Could you check a few things on this model? Use its own coordinates, in mm. Face numbers are marked on the shaded views. A direction names the side the tool comes from. Round coordinates to 2 decimals unless told otherwise and drop trailing zeros. Write each loop counter-clockwise with the first axis right and the second up, starting at its lowest first coordinate (ties: lowest second). Pieces come first, ordered by that corner, then holes. Notation, with made-up numbers: (34.25, 79.25) -> (39.25, 79.25) arc R23 ccw to (39.25, 109.25) -> close; hole circle Ø1 at (15.25, 81). An arc over 180 degrees is marked (long way). Answer in a Markdown table with one row per item. Add a question column.
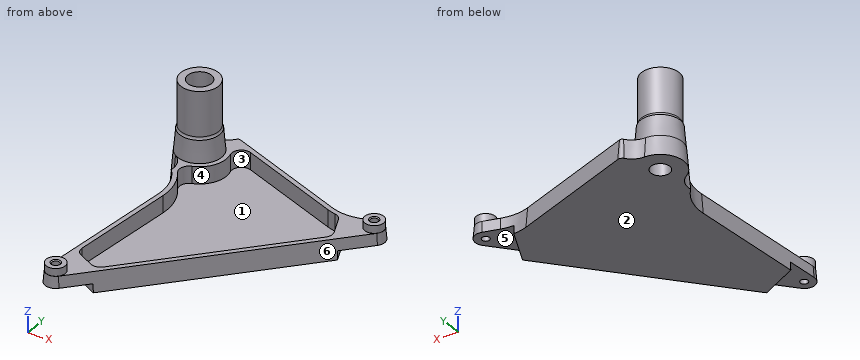
```python
from build123d import *
from build123d.topology import SkipClean

# Parameters (mm, degrees)
EXTRUDE_741_DEPTH      = 21
EXTRUDE_741_TAPER      = 5
SKETCH_2_R             = 10
EXTRUDE_1024_DEPTH     = 8
CUT_EXTRUDE_1617_DEPTH = 9
SKETCH_4_R             = 23.162738066
EXTRUDE_1852_DEPTH     = 23
EXTRUDE_1852_TAPER     = 5
SKETCH_5_R             = 20
EXTRUDE_1938_DEPTH     = 50
FILLET_1977_R          = 4
SKETCH_6_R             = 12.5
CUT_EXTRUDE_2083_DEPTH = 24
SKETCH_7_R             = 10
CUT_EXTRUDE_2165_DEPTH = 330.802615362
FILLET_2203_R          = 0.3
SKETCH_8_R             = 4
CUT_EXTRUDE_2369_DEPTH = 329.777683375
CHAMFER_2404_SIZE      = 1
CUT_EXTRUDE_3109_DEPTH = 18


with BuildPart() as part:
    # Эскиз1 → Extrude 741 (new body)
    with BuildSketch(Plane.XY):
        with BuildLine():
            ThreePointArc((206.902825712, -28.037707575), (208.16042902, -13.627270923), (194.643197369, -8.47686326))
            Line((194.643197369, -8.47686326), (178.352602864, -13.211762774))
            ThreePointArc((178.352602864, -13.211762774), (164.281318134, -14.974601832), (150.3601632, -12.270882024))
            Line((150.3601632, -12.270882024), (21.714759937, 34.696764669))
            ThreePointArc((21.714759937, 34.696764669), (18.576858011, 34.793189635), (16, 33))
            ThreePointArc((16, 33), (8.94427191, 27.11145618), (0, 25))
            ThreePointArc((0, 25), (-24.017605322, 6.939354046), (-13.333333333, -21.147629234))
            ThreePointArc((-13.333333333, -21.147629234), (-5.735545873, -29.916516988), (-4.284649798, -41.428018512))
            ThreePointArc((-4.284649798, -41.428018512), (6.155658081, -59.36704661), (8.411759167, -80))
            Line((8.411759167, -80), (-6.939849245, -232.746575098))
            ThreePointArc((-6.939849245, -232.746575098), (0.139115456, -244.91798346), (13.910401615, -241.984282673))
            Line((13.910401615, -241.984282673), (206.902825712, -28.037707575))
        make_face()
    extrude(amount=EXTRUDE_741_DEPTH, taper=EXTRUDE_741_TAPER)

    # Эскиз2 → Extrude 1024 (add)
    with BuildSketch(Plane.XY.offset(21)):
        with Locations((5, -233.946575098)):
            Circle(SKETCH_2_R)
        with Locations((197.992424097, -20)):
            Circle(SKETCH_2_R)
    extrude(amount=EXTRUDE_1024_DEPTH)

    # Эскиз3 → Cut-Extrude 1617 (cut)
    with BuildSketch(Plane(origin=(0, 0, 0), x_dir=(-1, 0, 0), z_dir=(0, 0, -1))):
        with BuildLine():
            Line((-164.992424097, -14.992878037), (-182.581248366, -55))
            Line((-182.581248366, -55), (-206.902825712, -28.037707575))
            ThreePointArc((-206.902825712, -28.037707575), (-208.364208989, -13.964597929), (-195.406790483, -8.281873067))
            Line((-195.406790483, -8.281873067), (-164.992424097, -14.992878037))
        make_face()
        with BuildLine():
            Line((3.643325211, -199.946575098), (-34.691772051, -218.946575098))
            Line((-34.691772051, -218.946575098), (-13.910401615, -241.984282673))
            ThreePointArc((-13.910401615, -241.984282673), (-0.139115456, -244.91798346), (6.939849245, -232.746575098))
            Line((6.939849245, -232.746575098), (3.643325211, -199.946575098))
        make_face()
    extrude(amount=-CUT_EXTRUDE_1617_DEPTH, mode=Mode.SUBTRACT)

    # Эскиз4 → Extrude 1852 (add)
    with SkipClean():  # the faces are left unmerged after this step: merging them gives an invalid solid
        with BuildSketch(Plane.XY.offset(21)):
            Circle(SKETCH_4_R)
        extrude(amount=EXTRUDE_1852_DEPTH, taper=EXTRUDE_1852_TAPER)

    # Эскиз5 → Extrude 1938 (add)
    with SkipClean():  # the faces are left unmerged after this step: merging them gives an invalid solid
        with BuildSketch(Plane.XY.offset(44)):
            Circle(SKETCH_5_R)
        extrude(amount=EXTRUDE_1938_DEPTH)

    # Fillet 1977
    # the kernel refuses this fillet: 4 mm, written as the material it adds along each edge
    with BuildSketch(Plane(origin=(0, 0, 44), x_dir=(1, 0, 0), z_dir=(0, -1, 0))) as fillet_1977_piece_1:
        with BuildLine():
            CenterArc((24, 2.807194852), FILLET_1977_R, 180, 44.571493735)
            Line((20, 2.807194852), (19.92, 2.807194852))
            Line((19.92, 2.807194852), (19.92, 0))
            Line((19.92, 0), (20, -0.08))
            ThreePointArc((20, -0.08), (20.575249402, -0.08), (21.093508781, -0.056143897))
            Line((21.093508781, -0.056143897), (21.150498805, 0))
        make_face()
    revolve(axis=Axis((0, 0, 44), (0, 0, 1)))

    # Эскиз6 → Cut-Extrude 2083 (cut)
    with SkipClean():  # the faces are left unmerged after this step: merging them gives an invalid solid
        with BuildSketch(Plane.XY.offset(94)):
            Circle(SKETCH_6_R)
        extrude(amount=-CUT_EXTRUDE_2083_DEPTH, mode=Mode.SUBTRACT)

    # Эскиз7 → Cut-Extrude 2165 (cut, through all)
    with SkipClean():  # the faces are left unmerged after this step: merging them gives an invalid solid
        with BuildSketch(Plane.XY.offset(70)):
            Circle(SKETCH_7_R)
        extrude(amount=-CUT_EXTRUDE_2165_DEPTH, mode=Mode.SUBTRACT)

    # Fillet 2203
    fillet_2203_edges = [part.edges().sort_by_distance(p)[0] for p in [
        (-10, 0, 70),
    ]]
    fillet(fillet_2203_edges, radius=FILLET_2203_R)

    # Эскиз8 → Cut-Extrude 2369 (cut, through all)
    with SkipClean():  # the faces are left unmerged after this step: merging them gives an invalid solid
        with BuildSketch(Plane.XY.offset(29)):
            with Locations((197.992424097, -20)):
                Circle(SKETCH_8_R)
            with Locations((5, -233.946575098)):
                Circle(SKETCH_8_R)
        extrude(amount=-CUT_EXTRUDE_2369_DEPTH, mode=Mode.SUBTRACT)

    # Chamfer 2404
    chamfer_2404_edges = [part.edges().sort_by_distance(p)[0] for p in [
        (193.992424097, -20, 29),
        (1, -233.946575098, 29),
    ]]
    chamfer(chamfer_2404_edges, length=CHAMFER_2404_SIZE)

    # Эскиз11 → Cut-Extrude 3109 (cut)
    with SkipClean():  # the faces are left unmerged after this step: merging them gives an invalid solid
        with BuildSketch(Plane.XY.offset(21)):
            with BuildLine():
                Line((9.637769662, -200.948644603), (25.017172577, -208.571128339))
                ThreePointArc((25.017172577, -208.571128339), (31.330335402, -209.434392448), (36.883287498, -206.3093368))
                Line((36.883287498, -206.3093368), (171.559935828, -57.010172388))
                ThreePointArc((171.559935828, -57.010172388), (174.007077586, -51.904002649), (173.288958057, -46.287439952))
                Line((173.288958057, -46.287439952), (164.797960407, -26.974018349))
                ThreePointArc((164.797960407, -26.974018349), (161.780560792, -23.10323492), (157.284911476, -21.134275293))
                ThreePointArc((157.284911476, -21.134275293), (152.593572172, -20.128602218), (148.015310631, -18.693484081))
                Line((148.015310631, -18.693484081), (39.848510542, 20.797550357))
                ThreePointArc((39.848510542, 20.797550357), (29.514566508, 18.6378946), (26.875914748, 8.415760323))
                ThreePointArc((26.875914748, 8.415760323), (25.216951873, -12.539742964), (9.508763983, -26.50892723))
                ThreePointArc((9.508763983, -26.50892723), (3.334586222, -32.957378734), (4.772476125, -41.76847801))
                ThreePointArc((4.772476125, -41.76847801), (13.557685978, -60.269741059), (15.214748896, -80.683726193))
                Line((15.214748896, -80.683726193), (4.128675533, -190.988763419))
                ThreePointArc((4.128675533, -190.988763419), (5.327976017, -196.828955218), (9.637769662, -200.948644603))
            make_face()
        extrude(amount=-CUT_EXTRUDE_3109_DEPTH, mode=Mode.SUBTRACT)


solid = part.part
```
(1) Suppose I cut it at D-D, the plane z = 60.5. Please give me the cut outline in (x, y), then the cut area to 3 significant figures.
(2) If we mould it in two halves opening along Y, with no side actions, what happens to the marked faces 3, 4, 5 and 6? For each: pulls with the +Y half, pulls with the -Y half, needs draft (parallel to the pull), parting line crosses it, or undercut.
(3) On a 3-axis mill with a long thin cutter (end or side, diameter ignored), from which of +Z, -Z, +X, -X, +Y, -Y can I reach the whole of each face in a straight line? I mean the marked faces 1 and 2. Say none if no direction works.
(4) I need wall thicknesses on L1, parallel to Y at x = 0, z = 48.5; L2, parallel to Y at x = 0, z = 84; L3, parallel to Z at x = 49, y = -39. Which ranges of each line are inside material? Lowest first, please.
(5) Suppose I cut it at B-B, the plane y = -110.5. Please give me the cut outline in (x, z).
(6) Suppose I cut it at A-A, the plane z = 74.5. Please give me the cut outline in (x, y).
(7) Suppose I cut it at C-C, the plane x = 52.5. Please give me the cut outline in (y, z).
(8) For P1, Ø10, axis at x = 5.5, y = -233.5, coming from the +Z side; P2, Ø6, axis at y = -12.5, z = 63.5, coming from the +X side; P3, Ø4, axis at y = -163, z = 19.5, coming from the +X side, each with a flat end and sliding along its axis, tell me the tip position at first contact or that it passes through.
Response:
| question | item | result |
|---|---|---|
| 1 | outline | circle Ø40 at (0, 0); hole circle Ø20 at (0, 0) |
| 1 | area | 942 mm² |
| 2 | face 3 | undercut |
| 2 | face 4 | undercut |
| 2 | face 5 | needs draft |
| 2 | face 6 | pulls with the -Y half |
| 3 | face 1 | +Z |
| 3 | face 2 | -Z, +X, -X, +Y, -Y |
| 4 | L1 | -20 to -10, 10 to 20 |
| 4 | L2 | -20 to -12.5, 12.5 to 20 |
| 4 | L3 | 0 to 3 |
| 5 | outline | (5.35, 0) -> (132.52, 0) -> (130.04, 21) -> (123.31, 21) -> (123.31, 3) -> (12.22, 3) -> (12.22, 21) -> (7.19, 21) -> close |
| 6 | outline | circle Ø40 at (0, 0); hole circle Ø25 at (0, 0) |
| 7 | outline | (-199.2, 0) -> (23.46, 0) -> (21.5, 21) -> (16.18, 21) -> (16.18, 3) -> (-189, 3) -> (-189, 21) -> (-196.46, 21) -> close |
| 8 | P1 | z = 29 |
| 8 | P2 | x = 17.6 |
| 8 | P3 | x = 84.68 |
